The listing builds one solid part. Answer for the finished solid, in the listing's coordinates (mm). Face numbers are marked on the shaded views. A direction names the side the tool comes from. Round coordinates to 2 decimals unless told otherwise and drop trailing zeros. Write each loop counter-clockwise with the first axis right and the second up, starting at its lowest first coordinate (ties: lowest second). Pieces come first, ordered by that corner, then holes.
(1) For the marked faces 1, 2 and 3, determine the directions among +Z, -Z, +X, -X, +Y, -Y from which every point of the face is accessible in a straight line to the end or side of a thin tool.
(2) Each of these flat-tipped pins is pushed along its axis until it touches: pin 1 Ø1 at (x, y) = (2.5, 1.5) entering from -Z; pin 2 Ø4 at (x, y) = (1.5, 9.5) entering from +Z. Where does it stop, or does it pass through?
(3) Find the intervals of material crossed by probe 1 along X at (y, z) = (8.25, 12); probe 2 along X at (y, z) = (11, 2.5); probe 3 along Y at (x, z) = (5.5, 3.75), in increasing order.
(4) A cutting plane is placed at B-B, the plane y = 2. Give the vertices of the cut face in (x, z), and give its area (3 significant figures).
(5) A cutting plane is placed at A-A, the plane z = 11.5. Give the vertices of the cut face in (x, y), and give its area (3 significant figures).
(6) A cutting plane is placed at D-D, the plane y = 13.75. Give the vertices of the cut face in (x, z), and give its area (3 significant figures).
(7) A cutting plane is placed at C-C, the plane x = 1.5. Give the vertices of the cut face in (y, z), and give its area (3 significant figures).
(8) The mould has two halves that part along Z. Classify the marked faces 4, 5, 6 and 7: +Z half, -Z half, draft (parallel to the pull), parting line (faces both ways), or undercut.
Autodesk Inventor part; units mm, degrees
ref_plane "YZ Plane" through (0, 0, 0) normal (1, 0, 0) x (0, 1, 0)
ref_plane "XZ Plane" through (0, 0, 0) normal (0, 1, 0) x (-1, 0, 0)
ref_plane "XY Plane" through (0, 0, 0) normal (0, 0, 1) x (1, 0, 0)
sketch "Sketch_1" plane through (0, 0, 0) normal (1, 0, 0) x (0, 1, 0)
  line L0 (0, 20) -> (0, 0)
  line L1 (0, 0) -> (20, 0)
  line L2 (20, 0) -> (20, 3)
  line L3 (20, 3) -> (3, 20)
  line L4 (3, 20) -> (0, 20)
  dimension "d35" = 20
  dimension "d36" = 20
  dimension "d37" = 17
  dimension "d38" = 3
extrude "Extrusion1" add sketch "Sketch_1" along normal mid plane 17
sketch "Sketch_2" plane through (0, 0, 0) normal (1, 0, 0) x (0, 1, 0)
  line L0 (3, 20) -> (3, 3.5)
  arc A0 (3, 3.5) -> (3.5, 3) centre (3.5, 3.5) ccw
  line L1 (3.5, 3) -> (20, 3)
  line L2 (20, 3) -> (3, 20)
extrude "Extrusion2" cut sketch "Sketch_2" along normal mid plane 13
sketch "Sketch_3" plane through (0, 0, 0) normal (1, 0, 0) x (0, 1, 0)
  line L0 (0, 3) -> (0, 0)
  line L1 (0, 0) -> (3, 0)
  line L2 (3, 0) -> (3, 1)
  line L3 (3, 1) -> (1, 1)
  line L4 (1, 1) -> (1, 3)
  line L5 (1, 3) -> (0, 3)
extrude "Extrusion3" cut sketch "Sketch_3" along normal mid plane 12
sketch "Sketch_4" plane through (0, 0, 0) normal (1, 0, 0) x (0, 1, 0)
  line L0 (0, 19) -> (0, 16)
  line L1 (0, 16) -> (1, 16)
  line L2 (1, 16) -> (1, 19)
  line L3 (1, 19) -> (0, 19)
extrude "Extrusion4" cut sketch "Sketch_4" along normal mid plane 12
sketch "Sketch_5" plane through (0, 0, 0) normal (1, 0, 0) x (0, 1, 0)
  line L0 (16, 1) -> (16, 0)
  line L1 (16, 0) -> (19, 0)
  line L2 (19, 0) -> (19, 1)
  line L3 (19, 1) -> (16, 1)
extrude "Extrusion5" cut sketch "Sketch_5" along normal mid plane 12
sketch "Sketch8" plane through (-8.5, 0, 20) normal (0, -1, 0) x (1, 0, 0)
  line L0 (8.5, -8) -> (8.5, -12) construction
  line L1 (5.75, -8) -> (5.75, -12)
  line L2 (11.25, -12) -> (11.25, -8)
  arc A0 (11.25, -8) -> (5.75, -8) centre (8.5, -8) ccw
  arc A1 (5.75, -12) -> (11.25, -12) centre (8.5, -12) ccw
  line L3 (14.5, -20) -> (2.5, -20)
  line L4 (17, 0) -> (17, -20)
  point P0 (8.5, -20)
  point P1 (8.5, -10)
  dimension "d23" = 2
  dimension "d24" = 5.5
  dimension "d25" = 10
  dimension "d32" = 8.5
extrude "Extrusion8" cut sketch "Sketch8" against normal through all
sketch "Sketch9" plane through (8.5, 20, 0) normal (0, 0, -1) x (-1, 0, 0)
  line L0 (8.5, -8) -> (8.5, -12) construction
  line L1 (5.75, -8) -> (5.75, -12)
  line L2 (11.25, -12) -> (11.25, -8)
  arc A0 (11.25, -8) -> (5.75, -8) centre (8.5, -8) ccw
  arc A1 (5.75, -12) -> (11.25, -12) centre (8.5, -12) ccw
  line L3 (17, -20) -> (14.5, -20)
  line L4 (0, -20) -> (0, 0)
  point P0 (8.5, -20)
  point P1 (8.5, -10)
  dimension "d28" = 2
  dimension "d29" = 5.5
  dimension "d30" = 10
  dimension "d31" = 8.5
extrude "Extrusion9" cut sketch "Sketch9" against normal through all
properties part number "14056_m"
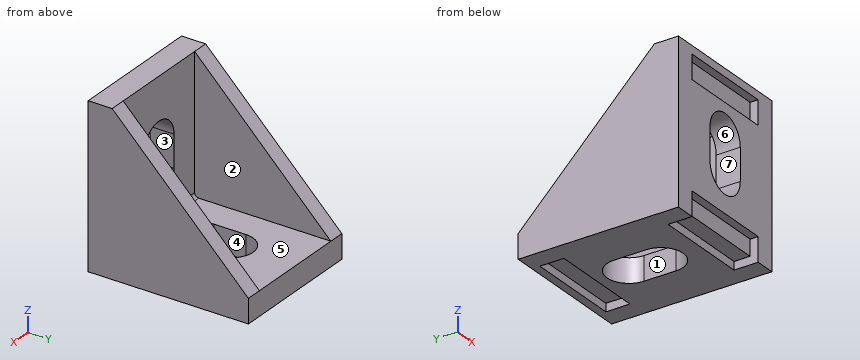
Solutions:
1. face 1: +Z, -Z
1. face 2: +Z, +Y
1. face 3: +Y, -Y
2. pin 1: stops at z = 1
2. pin 2: stops at z = 3
3. probe 1: x = -8.5 to -6.5, 6.5 to 8.5
3. probe 2: x = -8.5 to -2.75, 2.75 to 8.5
3. probe 3: y = 0 to 3
4. outline: (-8.5, 0) - (-6, 0) - (-6, 1) - (6, 1) - (6, 0) - (8.5, 0) - (8.5, 20) - (-8.5, 20) - close; hole (-2.75, 8) arc R2.75 ccw to (2.75, 8) - (2.75, 12) arc R2.75 ccw to (-2.75, 12) - close
4. area: 282 mm2
5. outline: (-8.5, 0) - (-2.75, 0) - (-2.75, 3) - (-6.5, 3) - (-6.5, 11.5) - (-8.5, 11.5) - close; (2.75, 0) - (8.5, 0) - (8.5, 11.5) - (6.5, 11.5) - (6.5, 3) - (2.75, 3) - close
5. area: 68.5 mm2
6. outline: (-8.5, 0) - (-2.12, 0) - (-2.12, 3) - (-6.5, 3) - (-6.5, 9.25) - (-8.5, 9.25) - close; (2.12, 0) - (8.5, 0) - (8.5, 9.25) - (6.5, 9.25) - (6.5, 3) - (2.12, 3) - close
6. area: 63.3 mm2
7. outline: (0, 3) - (1, 3) - (1, 1) - (3, 1) - (3, 0) - (5.7, 0) - (5.7, 3) - (3.5, 3) arc R0.5 cw to (3, 3.5) - (3, 5.7) - (0, 5.7) - close; (0, 14.3) - (3, 14.3) - (3, 20) - (0, 20) - (0, 19) - (1, 19) - (1, 16) - (0, 16) - close; (14.3, 0) - (16, 0) - (16, 1) - (19, 1) - (19, 0) - (20, 0) - (20, 3) - (14.3, 3) - close
7. area: 48.4 mm2
8. face 4: draft
8. face 5: +Z half
8. face 6: undercut
8. face 7: undercut
